Geometry: final body of the model. Coordinates: model frame, mm. A direction names the side the tool comes from. Give positions to 0.01 mm unless a question says otherwise; leave off trailing zeros. Loops run counter-clockwise (first coordinate to the right, second up) from the corner with the lowest first, then second, coordinate; pieces in that order, holes last. Notation, with made-up numbers: M -0.5,-23 L 8.5,-23 A8 ccw 8.5,-10 Z; hole C 22,46 d5. An arc over 180 degrees is marked long. Put each result on its own line as item: value.
```python
from build123d import *

# Parameters (mm, degrees)
BOSS_EXTRUDE1_DEPTH = 5.9
SKETCH2_R           = 0.3
BOSS_EXTRUDE2_DEPTH = 3.5
SKETCH3_R           = 0.3
CUT_EXTRUDE1_DEPTH  = 3.5


with BuildPart() as part:
    # Sketch1 → Boss-Extrude1 (new body)
    with BuildSketch(Plane(origin=(0, 0, 0), x_dir=(1, 0, 0), z_dir=(0, 1, 0))):
        Polygon((-4.2, 2.45), (-4.95, 1.7), (-4.95, -2.45), (4.95, -2.45), (4.95, 2.45), align=None)
    extrude(amount=-BOSS_EXTRUDE1_DEPTH)

    # Sketch2 → Boss-Extrude2 (add)
    with BuildSketch(Plane.XZ.offset(5.9)):
        with Locations(Location((-2.5, 0, 0), (0, 0, 90))):
            Circle(SKETCH2_R)
        with Locations(Location((-0.05, 0, 0), (0, 0, 90))):
            Circle(SKETCH2_R)
        with Locations(Location((2.4, 0, 0), (0, 0, 90))):
            Circle(SKETCH2_R)
    extrude(amount=BOSS_EXTRUDE2_DEPTH)

    # Sketch3 → Cut-Extrude1 (cut)
    with BuildSketch(Plane(origin=(0, 0, 0), x_dir=(1, 0, 0), z_dir=(0, 1, 0))):
        Polygon((-1.603247496, 1.75), (-3.5, 1.75), (-4.25, 1), (-4.25, -0.65), (-4.95, -0.65), (-4.95, -1.25), (-4.25, -1.25), (-4.25, -1.75), (4.25, -1.75), (4.25, -1.25), (4.95, -1.25), (4.95, -0.65), (4.25, -0.65), (4.25, 1), (3.5, 1.75), (1.503247496, 1.75), (1.175, 1.421752504), (0.846752504, 1.75), (-0.946752504, 1.75), (-1.275, 1.421752504), align=None)
        with Locations(Location((-2.5, 0.63, 0), (0, 0, 270))):
            Circle(SKETCH3_R, mode=Mode.SUBTRACT)
        with Locations(Location((-0.05, 0.63, 0), (0, 0, 270))):
            Circle(SKETCH3_R, mode=Mode.SUBTRACT)
        with Locations(Location((2.4, 0.63, 0), (0, 0, 270))):
            Circle(SKETCH3_R, mode=Mode.SUBTRACT)
    extrude(amount=-CUT_EXTRUDE1_DEPTH, mode=Mode.SUBTRACT)


solid = part.part
```
Item 1: Section A-A on y = -2.5. Output: boundary loops of the cut face in (x, z) (3 decimals), then the cut area to 3 significant figures.
Output values:
outline: M -4.95,-1.7 L -4.2,-2.45 L 4.95,-2.45 L 4.95,0.65 L 4.25,0.65 L 4.25,-1 L 3.5,-1.75 L 1.503,-1.75 L 1.175,-1.422 L 0.847,-1.75 L -0.947,-1.75 L -1.275,-1.422 L -1.603,-1.75 L -3.5,-1.75 L -4.25,-1 L -4.25,0.65 L -4.95,0.65 Z; M -4.95,1.25 L -4.25,1.25 L -4.25,1.75 L 4.25,1.75 L 4.25,1.25 L 4.95,1.25 L 4.95,2.45 L -4.95,2.45 Z; C -2.5,-0.63 d0.6; C -0.05,-0.63 d0.6; C 2.4,-0.63 d0.6
area: 19.3 mm²
Item 2: Line query: probe 1 along Z at (x, y) = (3.25, -1.25); probe 2 along X at (y, z) = (-8.5, -0.15); probe 3 along Y at (x, z) = (-2.75, -1.45). Output: solid intervals per line, ascending. Write a range as [from, to].
Output values:
probe 1: [-2.45, -1.75], [1.75, 2.45]
probe 2: [-2.76, -2.24], [-0.31, 0.21], [2.14, 2.66]
probe 3: [-5.9, -3.5]
Item 3: Pin query (flat end, axial travel): pin 1 Ø1 at (x, z) = (-2.5, 1) entering from +Y; pin 2 Ø1.5 at (y, z) = (-8.5, 1.5) entering from +X. Return the tip coordinate at first contact, or that it passes through.
Output values:
pin 1: y = -3.5
pin 2: through
Item 4: Section D-D on z = -0.8. Output: boundary loops of the cut face in (x, y).
Output values:
outline: M -4.95,-5.9 L 4.95,-5.9 L 4.95,0 L 4.25,0 L 4.25,-3.5 L 2.65,-3.5 L 2.65,0 L 2.15,0 L 2.15,-3.5 L 0.2,-3.5 L 0.2,0 L -0.3,0 L -0.3,-3.5 L -2.25,-3.5 L -2.25,0 L -2.75,0 L -2.75,-3.5 L -4.25,-3.5 L -4.25,0 L -4.95,0 Z
Item 5: Set-up query: faces 5 (the flat face through (0, -2, 1.75)), 6 (the flat face through (0, 0, 2)). Return all of +Z, -Z, +X, -X, +Y, -Y with unobstructed straight access to the full face (end or side cutting, diameter ignored); none if empty.
Output values:
face 5: +Y
face 6: +Z, -Z, +X, -X, +Y
Item 6: Section C-C on x = -2.5. Output: boundary loops of the cut face in (y, z), then the cut area to 3 significant figures.
Output values:
outline: M -9.4,-0.3 L -5.9,-0.3 L -5.9,-2.45 L 0,-2.45 L 0,-1.75 L -3.5,-1.75 L -3.5,-0.93 L 0,-0.93 L 0,-0.33 L -3.5,-0.33 L -3.5,1.75 L 0,1.75 L 0,2.45 L -5.9,2.45 L -5.9,0.3 L -9.4,0.3 Z
area: 20.9 mm²
Item 7: Mould query, pull axis Z, two halves, no side actions, for faces 1 (the flat face through (0, -3, -2.45)), 2 (the flat face through (4.95, -3, 0)), 3 (the flat face through (-3, -2, -1.75)), 4 (the flat face through (0, -2, -1.75)). Classes: pulls with the +Z half, pulls with the -Z half, needs draft (parallel to the pull), parting line crosses it, or undercut.
Output values:
face 1: pulls with the -Z half
face 2: needs draft
face 3: undercut
face 4: undercut
Item 8: Section B-B on z = 1.45. Output: boundary loops of the cut face in (x, y).
Output values:
outline: M -4.95,-5.9 L 4.95,-5.9 L 4.95,0 L 4.25,0 L 4.25,-3.5 L -4.25,-3.5 L -4.25,0 L -4.95,0 Z
